Part model, mm, in its own coordinate system. Face numbers are marked on the shaded views. Coordinates: 2 decimals unless noted, no trailing zeros. Use a Markdown table: item, result. Add a question column.
1. Band-saw the part on A-A, the plane x = 0. Count the separate pieces of the cut face and the enclosed holes in it, plus the area to 3 significant figures.
2. Pull direction X, two halves, no side cores. Call the marked faces 1 and 2: pulls with the +X half, pulls with the -X half, needs draft (parallel to the pull), parting line crosses it, or undercut.
3. Wall check: probe 1 along Y at (x, z) = (0, 2.1); probe 2 along Y at (x, z) = (30, 1.2); probe 3 along Z at (x, y) = (44.5, 1). Give the ranges that are in metal, low to high. Write a range as [from, to].
4. Drop flat-ended pins along their axis: pin 1 (1.5 mm diameter, centred on x = 3, z = 1.5, fed in from -Y); pin 2 (1.5 mm diameter, centred on x = 7.78, y = 7.78, fed in from +Z); pin 3 (3 mm diameter, centred on y = 14.5, z = 1, fed in from +X); pin 4 (3 mm diameter, centred on x = 0, y = 11, fed in from -Z). Give the stop position or say it passes through.
from build123d import *

# Parameters (mm, degrees)
SKETCH_1_R            = 50
EXTRUDE_1_DEPTH       = 3
F_2_5MM_1_D           = 2.5
F_2_5MM_1_CSINK_D     = 2.55
F_2_5MM_1_CSINK_ANGLE = 90
SKETCH_5_R            = 20
EXTRUDE_2_DEPTH       = 3
SKETCH_6_R            = 17
CUT_EXTRUDE_1_DEPTH   = 5
F_2_5MM_2_AT_2_COUNT  = 2
F_2_5MM_2_AT_2_PITCH  = 8.419035512
F_2_5MM_2_AT_3_COUNT  = 2
F_2_5MM_2_AT_3_PITCH  = 15.556349186
F_2_5MM_2_AT_4_COUNT  = 2
F_2_5MM_2_AT_4_PITCH  = 20.325349715
F_2_5MM_2_AT_5_COUNT  = 2
F_2_5MM_2_AT_5_PITCH  = 22
F_2_5MM_2_AT_6_COUNT  = 2
F_2_5MM_2_AT_6_PITCH  = 20.325349715
F_2_5MM_2_AT_7_COUNT  = 2
F_2_5MM_2_AT_7_PITCH  = 15.556349186
F_2_5MM_2_AT_8_COUNT  = 2
F_2_5MM_2_AT_8_PITCH  = 8.419035512
SKETCH_10_R           = 5
CUT_EXTRUDE_2_DEPTH   = 5
FILLET_1_R            = 1
FILLET_3_R            = 3


# Some blends are built 0.0001 mm under size
with BuildPart() as part:
    # 草图1 → 凸台-拉伸1 (new body)
    with BuildSketch(Plane.XY):
        Circle(SKETCH_1_R)
    extrude(amount=EXTRUDE_1_DEPTH)

    # Ø2.5mm 暗销孔1 (through all)
    with Locations(Plane(origin=(0, 0, 0), x_dir=(-1, 0, 0), z_dir=(0, 0, -1))):
        with Locations((-30, 10), (-30, -10), (30, -10), (30, 10)):
            CounterSinkHole(F_2_5MM_1_D / 2, F_2_5MM_1_CSINK_D / 2, counter_sink_angle=F_2_5MM_1_CSINK_ANGLE)

    # 草图5 → 凸台-拉伸2 (add)
    with BuildSketch(Plane.XY.offset(3)):
        Circle(SKETCH_5_R)
    extrude(amount=EXTRUDE_2_DEPTH)

    # 草图6 → 切除-拉伸1 (cut)
    with BuildSketch(Plane(origin=(0, 0, 0), x_dir=(-1, 0, 0), z_dir=(0, 0, -1))):
        Circle(SKETCH_6_R)
    extrude(amount=-CUT_EXTRUDE_1_DEPTH, mode=Mode.SUBTRACT)

    # 草图9 → Ø2.5mm 暗销孔2 (revolve, cut)
    with BuildSketch(Plane(origin=(11, 0, 5), x_dir=(0, 1, 0), z_dir=(1, 0, 0))):
        Polygon((0, 0), (0, 1), (1.25, 1), (1.25, 0.025), (1.275, 0), align=None)
    f_2_5mm_2 = revolve(axis=Axis((11, 0, -1.35), (0, 0, 1)), mode=Mode.SUBTRACT)

    # Ø2.5mm 暗销孔2 at 2: Ø2.5mm 暗销孔2 ×2
    with Locations(*[Vector(-0.38268343236200486, 0.9238795325125646, 0) * (i * F_2_5MM_2_AT_2_PITCH) for i in range(1, F_2_5MM_2_AT_2_COUNT)]):
        add(f_2_5mm_2, mode=Mode.SUBTRACT)

    # Ø2.5mm 暗销孔2 at 3: Ø2.5mm 暗销孔2 ×2
    with Locations(*[Vector(-0.7071067811841869, 0.7071067811889081, 0) * (i * F_2_5MM_2_AT_3_PITCH) for i in range(1, F_2_5MM_2_AT_3_COUNT)]):
        add(f_2_5mm_2, mode=Mode.SUBTRACT)

    # Ø2.5mm 暗销孔2 at 4: Ø2.5mm 暗销孔2 ×2
    with Locations(*[Vector(-0.9238795325100095, 0.3826834323681732, 0) * (i * F_2_5MM_2_AT_4_PITCH) for i in range(1, F_2_5MM_2_AT_4_COUNT)]):
        add(f_2_5mm_2, mode=Mode.SUBTRACT)

    # Ø2.5mm 暗销孔2 at 5: Ø2.5mm 暗销孔2 ×2
    with Locations(*[(-i * F_2_5MM_2_AT_5_PITCH, 0, 0) for i in range(1, F_2_5MM_2_AT_5_COUNT)]):
        add(f_2_5mm_2, mode=Mode.SUBTRACT)

    # Ø2.5mm 暗销孔2 at 6: Ø2.5mm 暗销孔2 ×2
    with Locations(*[Vector(-0.9238795325125633, -0.38268343236200797, 0) * (i * F_2_5MM_2_AT_6_PITCH) for i in range(1, F_2_5MM_2_AT_6_COUNT)]):
        add(f_2_5mm_2, mode=Mode.SUBTRACT)

    # Ø2.5mm 暗销孔2 at 7: Ø2.5mm 暗销孔2 ×2
    with Locations(*[Vector(-0.7071067811889058, -0.7071067811841893, 0) * (i * F_2_5MM_2_AT_7_PITCH) for i in range(1, F_2_5MM_2_AT_7_COUNT)]):
        add(f_2_5mm_2, mode=Mode.SUBTRACT)

    # Ø2.5mm 暗销孔2 at 8: Ø2.5mm 暗销孔2 ×2
    with Locations(*[Vector(-0.3826834323681702, -0.9238795325100109, 0) * (i * F_2_5MM_2_AT_8_PITCH) for i in range(1, F_2_5MM_2_AT_8_COUNT)]):
        add(f_2_5mm_2, mode=Mode.SUBTRACT)

    # 草图10 → 切除-拉伸2 (cut)
    with BuildSketch(Plane(origin=(0, 0, 5), x_dir=(-1, 0, 0), z_dir=(0, 0, -1))):
        Circle(SKETCH_10_R)
    extrude(amount=-CUT_EXTRUDE_2_DEPTH, mode=Mode.SUBTRACT)

    # 圆角1
    # the kernel refuses this fillet: 1 mm, written as the material it takes off along each edge
    with BuildSketch(Plane(origin=(-30, -10, 0), x_dir=(1, 0, 0), z_dir=(0, -1, 0))) as fillet_1_piece_1:
        with BuildLine():
            CenterArc((1.47220486, 1), FILLET_1_R, 257.161431859, 12.838568141)
            Line((1.25, 0.025), (1.245555903, 0.0055))
            ThreePointArc((1.245555903, 0.0055), (1.248357864, -0.001642136), (1.260857864, -0.014142136))
            Line((1.260857864, -0.014142136), (1.275, -0.02))
            Line((1.275, -0.02), (1.47220486, -0.02))
            Line((1.47220486, -0.02), (1.47220486, 0))
        make_face()
    revolve(axis=Axis((-30, -10, 0), (0, 0, 1)), mode=Mode.SUBTRACT)
    with BuildSketch(Plane(origin=(0, 0, 0), x_dir=(1, 0, 0), z_dir=(0, -1, 0))) as fillet_1_piece_2:
        with BuildLine():
            CenterArc((50 - FILLET_1_R, FILLET_1_R), FILLET_1_R, 270, 90)
            Line((50 - FILLET_1_R, 0), (50 - FILLET_1_R, -FILLET_1_R * 0.02))
            Line((50 - FILLET_1_R, -FILLET_1_R * 0.02), (50 + FILLET_1_R * 0.02, -FILLET_1_R * 0.02))
            Line((50 + FILLET_1_R * 0.02, -FILLET_1_R * 0.02), (50 + FILLET_1_R * 0.02, FILLET_1_R))
            Line((50 + FILLET_1_R * 0.02, FILLET_1_R), (50, FILLET_1_R))
        make_face()
    revolve(axis=Axis((0, 0, 0), (0, 0, 1)), mode=Mode.SUBTRACT)
    with BuildSketch(Plane(origin=(30, -10, 0), x_dir=(1, 0, 0), z_dir=(0, -1, 0))) as fillet_1_piece_3:
        with BuildLine():
            CenterArc((1.47220486, 1), FILLET_1_R, 257.161431859, 12.838568141)
            Line((1.25, 0.025), (1.245555903, 0.0055))
            ThreePointArc((1.245555903, 0.0055), (1.248357864, -0.001642136), (1.260857864, -0.014142136))
            Line((1.260857864, -0.014142136), (1.275, -0.02))
            Line((1.275, -0.02), (1.47220486, -0.02))
            Line((1.47220486, -0.02), (1.47220486, 0))
        make_face()
    revolve(axis=Axis((30, -10, 0), (0, 0, 1)), mode=Mode.SUBTRACT)
    with BuildSketch(Plane(origin=(30, 10, 0), x_dir=(1, 0, 0), z_dir=(0, -1, 0))) as fillet_1_piece_4:
        with BuildLine():
            CenterArc((1.47220486, 1), FILLET_1_R, 257.161431859, 12.838568141)
            Line((1.25, 0.025), (1.245555903, 0.0055))
            ThreePointArc((1.245555903, 0.0055), (1.248357864, -0.001642136), (1.260857864, -0.014142136))
            Line((1.260857864, -0.014142136), (1.275, -0.02))
            Line((1.275, -0.02), (1.47220486, -0.02))
            Line((1.47220486, -0.02), (1.47220486, 0))
        make_face()
    revolve(axis=Axis((30, 10, 0), (0, 0, 1)), mode=Mode.SUBTRACT)
    with BuildSketch(Plane(origin=(0, 0, 0), x_dir=(-1, 0, 0), z_dir=(0, -1, 0))) as fillet_1_piece_5:
        with BuildLine():
            CenterArc((17 + FILLET_1_R, -FILLET_1_R), FILLET_1_R, 90, 90)
            Line((17, -FILLET_1_R), (17 - FILLET_1_R * 0.02, -FILLET_1_R))
            Line((17 - FILLET_1_R * 0.02, -FILLET_1_R), (17 - FILLET_1_R * 0.02, FILLET_1_R * 0.02))
            Line((17 - FILLET_1_R * 0.02, FILLET_1_R * 0.02), (17 + FILLET_1_R, FILLET_1_R * 0.02))
            Line((17 + FILLET_1_R, FILLET_1_R * 0.02), (17 + FILLET_1_R, 0))
        make_face()
    revolve(axis=Axis((0, 0, 0), (0, 0, -1)), mode=Mode.SUBTRACT)
    with BuildSketch(Plane(origin=(-30, 10, 0), x_dir=(1, 0, 0), z_dir=(0, -1, 0))) as fillet_1_piece_6:
        with BuildLine():
            CenterArc((1.47220486, 1), FILLET_1_R, 257.161431859, 12.838568141)
            Line((1.25, 0.025), (1.245555903, 0.0055))
            ThreePointArc((1.245555903, 0.0055), (1.248357864, -0.001642136), (1.260857864, -0.014142136))
            Line((1.260857864, -0.014142136), (1.275, -0.02))
            Line((1.275, -0.02), (1.47220486, -0.02))
            Line((1.47220486, -0.02), (1.47220486, 0))
        make_face()
    revolve(axis=Axis((-30, 10, 0), (0, 0, 1)), mode=Mode.SUBTRACT)

    # 圆角3
    fillet_3_edges = [part.edges().sort_by_distance(p)[0] for p in [
        (-20, 0, 3),
    ]]
    fillet(fillet_3_edges, radius=FILLET_3_R - 0.0001)  # a hair under: the kernel refuses the full size


solid = part.part
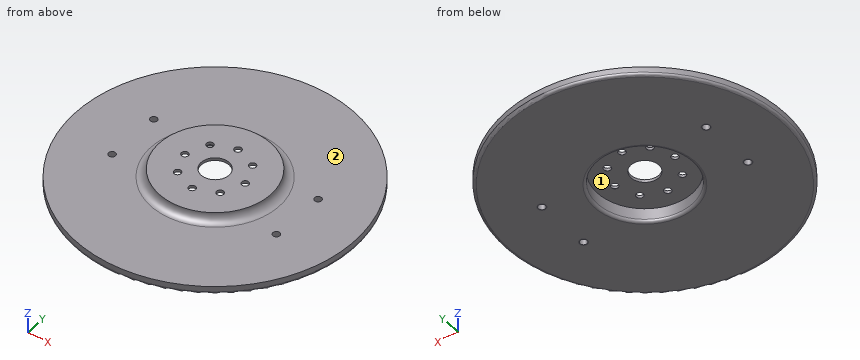
Geometry check:
| question | item | result |
|---|---|---|
| 1 | separate pieces | 4 |
| 1 | enclosed holes | 0 |
| 1 | area | 238 mm^2 |
| 2 | face 1 | undercut |
| 2 | face 2 | needs draft |
| 3 | probe 1 | y = [-50, -17], [17, 50] |
| 3 | probe 2 | y = [-40, -11.25], [-8.75, 8.75], [11.25, 40] |
| 3 | probe 3 | z = [0, 3] |
| 4 | pin 1 | stops at y = -49.95 |
| 4 | pin 2 | passes through |
| 4 | pin 3 | stops at x = 48.28 |
| 4 | pin 4 | stops at z = 5 |
